The listing builds one solid part. Answer for the finished solid, in the listing's coordinates (mm). A direction names the side the tool comes from. Coordinates: 2 decimals unless noted, no trailing zeros. Order: outer loops, then holes, each group sorted by start corner. A loop starts at its lowest first (then second) coordinate and runs counter-clockwise, first axis right, second up. Notation, with made-up numbers: (64, 28) -> (122, 28) arc R20 ccw to (122, 49) -> close; hole circle Ø9 at (-19, 78). An arc over 180 degrees is marked (long way). Return JSON: item names as keys, results as strings.
from build123d import *

# Parameters (mm, degrees)
F0_R     = 25.4
F1_DEPTH = 10.16
F2_SIZE  = 5.08
F3_R     = 2.54
F4_DEPTH = 10.161
F5_R     = 1.524
F6_DEPTH = 10.161
F8_DEPTH = 3.81


with BuildPart() as f1:
    # F0 (on Top) → F1 (new body)
    with BuildSketch(Plane.XY):
        Circle(F0_R)
    extrude(amount=F1_DEPTH)

    # F2
    f2_edges = [f1.edges().sort_by_distance(p)[0] for p in [
        (-25.4, 0, 10.16),
    ]]
    chamfer(f2_edges, length=F2_SIZE)

    # F3 (on face) → F4 (cut, through all)
    with BuildSketch(Plane.XY.offset(10.16)):
        Circle(F3_R)
    extrude(amount=-F4_DEPTH, mode=Mode.SUBTRACT)

    # F5 (on face) → F6 (cut, through all)
    with BuildSketch(Plane.XY.offset(10.16)):
        with Locations((-8.980256, -8.980256)):
            Circle(F5_R)
        with Locations((8.980256, -8.980256)):
            Circle(F5_R)
        with Locations((0, 12.7)):
            Circle(F5_R)
        with Locations((-8.980256, 8.980256)):
            Circle(F5_R)
        with Locations((-12.7, 0)):
            Circle(F5_R)
        with Locations((12.7, 0)):
            Circle(F5_R)
        with Locations((8.980256, 8.980256)):
            Circle(F5_R)
        with Locations((0, -12.7)):
            Circle(F5_R)
    extrude(amount=-F6_DEPTH, mode=Mode.SUBTRACT)

    # F7 (on face) → F8 (cut)
    with BuildSketch(Plane.XY.offset(10.16)):
        with BuildLine():
            Line((23.970625, 2.54), (20.160625, 2.54))
            ThreePointArc((20.160625, 2.54), (17.775005, 0), (20.160625, -2.54))
            Line((20.160625, -2.54), (23.970625, -2.54))
            Line((23.970625, -2.54), (23.970625, 2.54))
        make_face()
        with BuildLine():
            Line((-2.54, 23.970625), (-2.54, 20.160625))
            ThreePointArc((-2.54, 20.160625), (0, 17.775005), (2.54, 20.160625))
            Line((2.54, 20.160625), (2.54, 23.970625))
            Line((2.54, 23.970625), (-2.54, 23.970625))
        make_face()
        with BuildLine():
            Line((-23.970625, -2.54), (-20.160625, -2.54))
            ThreePointArc((-20.160625, -2.54), (-17.775005, 0), (-20.160625, 2.54))
            Line((-20.160625, 2.54), (-23.970625, 2.54))
            Line((-23.970625, 2.54), (-23.970625, -2.54))
        make_face()
        with BuildLine():
            Line((2.54, -23.970625), (2.54, -20.160625))
            ThreePointArc((2.54, -20.160625), (0, -17.775005), (-2.54, -20.160625))
            Line((-2.54, -20.160625), (-2.54, -23.970625))
            Line((-2.54, -23.970625), (2.54, -23.970625))
        make_face()
    extrude(amount=-F8_DEPTH, mode=Mode.SUBTRACT)


solid = f1.part
1. The part is cut by section A-A on x = 0. Give the vertices of the cut face in (y, z) (3 decimals).
Answer block:
{"outline": "(-25.4, 0) -> (-14.224, 0) -> (-14.224, 10.16) -> (-17.775, 10.16) -> (-17.775, 6.35) -> (-23.971, 6.35) -> (-23.971, 6.509) -> (-25.4, 5.08) -> close; (-11.176, 0) -> (-2.54, 0) -> (-2.54, 10.16) -> (-11.176, 10.16) -> close; (2.54, 0) -> (11.176, 0) -> (11.176, 10.16) -> (2.54, 10.16) -> close; (14.224, 0) -> (25.4, 0) -> (25.4, 5.08) -> (23.971, 6.509) -> (23.971, 6.35) -> (17.775, 6.35) -> (17.775, 10.16) -> (14.224, 10.16) -> close"}
2. For faces 1 (the face through (21, 0, 6.35)), 2 (the face through (-0.33, -14.188, 5.151)), determine the directions among +Z, -Z, +X, -X, +Y, -Y from which every point of the face is accessible in a straight line to the end or side of a thin tool.
Answer block:
{"face 1": "+Z", "face 2": "+Z, -Z"}
3. Each of these flat-tipped pins is pushed along its axis until it touches: pin 1 Ø6 at (y, z) = (11, 1.5) entering from +X; pin 2 Ø5 at (x, z) = (-18, 2) entering from +Y; pin 3 Ø6 at (x, z) = (5, 5) entering from +Y. Where does it stop, or does it pass through?
Answer block:
{"pin 1": "stops at x = 24.11", "pin 2": "stops at y = 20.12", "pin 3": "stops at y = 25.32"}
4. Determine the mould class of faces 3 (the face through (-5.506, -24.796, 2.504)), 4 (the face through (22, -2.54, 8)), 5 (the face through (5, 0, 0)) for opening direction Y: pulls with the +Y half, pulls with the -Y half, needs draft (parallel to the pull), parting line crosses it, or undercut.
Answer block:
{"face 3": "parting line crosses it", "face 4": "undercut", "face 5": "needs draft"}
5. The part is cut by section C-C on z = 2.75. Give the number of separate pieces and of enclosed holes in the cut face, and give its area (3 significant figures).
Answer block:
{"separate pieces": "1", "enclosed holes": "9", "area": "1,950 mm2"}
6. Consider line 1 (Y direction, x = 0, z = 5); line 2 (Y direction, x = 0, z = 7.75) (3 decimals); line 3 (X direction, y = 10, z = 7.5). Determine where each line is inside the solid, lowest interval first. Write a range as from..to.
Answer block:
{"line 1": "y = -25.4..-14.22, -11.18..-2.54, 2.54..11.18, 14.22..25.4", "line 2": "y = -17.775..-14.224, -11.176..-2.54, 2.54..11.176, 14.224..17.775", "line 3": "x = -20.69..-10.11, -7.85..7.85, 10.11..20.69"}
